from build123d import *

# Parameters (mm, degrees)
SKETCH1_R           = 5.584000144
BOSS_EXTRUDE1_DEPTH = 15
SKETCH2_R           = 2.6
CUT_EXTRUDE1_DEPTH  = 8.2
SKETCH3_R           = 2.55
CUT_EXTRUDE2_DEPTH  = 7


with BuildPart() as part:
    # Sketch1 → Boss-Extrude1 (new body)
    with BuildSketch(Plane.XY):
        with Locations((-60.533127818, -24.469533588)):
            Circle(SKETCH1_R)
    extrude(amount=BOSS_EXTRUDE1_DEPTH)

    # Sketch2 → Cut-Extrude1 (cut)
    with BuildSketch(Plane(origin=(0, 0, 0), x_dir=(-1, 0, 0), z_dir=(0, 0, -1))):
        with Locations((60.533127818, -24.469533588)):
            Circle(SKETCH2_R)
    extrude(amount=-CUT_EXTRUDE1_DEPTH, mode=Mode.SUBTRACT)

    # Sketch3 → Cut-Extrude2 (cut)
    with BuildSketch(Plane.XY.offset(15)):
        with Locations((-60.533127818, -24.469533588)):
            Circle(SKETCH3_R)
    extrude(amount=-CUT_EXTRUDE2_DEPTH, mode=Mode.SUBTRACT)


solid = part.part
Verification items for the finished model (mm, model axes). Give positions to 0.01 mm unless a question says otherwise; leave off trailing zeros. Loops run counter-clockwise (first coordinate to the right, second up) from the corner with the lowest first, then second, coordinate; pieces in that order, holes last.
1) Sectioned sample at D-D, the plane y = -19.75. Enter the section's corners in (x, z), then the cut area to 3 significant figures.
2) Draft check along Y on faces 1 (the flat face through (-58, -26, 0)), 2 (the cylindrical face through (-61.74, -29.92, 7.4)), 3 (the cylindrical face through (-58.62, -22.71, 4.04)). Enter one of: pulls with the +Y half, pulls with the -Y half, needs draft (parallel to the pull), parting line crosses it, or undercut.
3) Sectioned sample at A-A, the plane x = -59.25. Enter the section's corners in (y, z), then the cut area to 3 significant figures.
4) Depth check by flat-ended pin: pin 1 Ø3 at (x, z) = (-58.5, 2.5) entering from +Y; pin 2 Ø1 at (x, z) = (-63.5, 2.5) entering from -Y; pin 3 Ø2 at (x, z) = (-58.5, 13.5) entering from +Y; pin 4 Ø6.5 at (x, y) = (-60.53, -24.47) entering from -Z. Enter the tip coordinate at first touch or a pass-through.
5) Thickness scan on line 1 along Y through (x, z) = (-60.5, 11.25); line 2 along X through (y, z) = (-26, 3.5); line 3 along Y through (x, z) = (-61.5, 5.5). Record the ranges inside material, lowest first.
6) Sectioned sample at C-C, the plane z = 10. Enter the section's corners in (x, y).
7) Sectioned sample at B-B, the plane y = -26.5. Enter the section's corners in (x, z), then the cut area to 3 significant figures.
Answers:
1. outline: (-63.52, 0) - (-57.55, 0) - (-57.55, 15) - (-63.52, 15) - close
1. area: 89.5 mm2
2. face 1: needs draft
2. face 2: parting line crosses it
2. face 3: undercut
3. outline: (-29.9, 0) - (-26.73, 0) - (-26.73, 8.2) - (-26.67, 8.2) - (-26.67, 15) - (-29.9, 15) - close; (-22.27, 8.2) - (-22.21, 8.2) - (-22.21, 0) - (-19.03, 0) - (-19.03, 15) - (-22.27, 15) - close
3. area: 96.0 mm2
4. pin 1: stops at y = -18.91
4. pin 2: stops at y = -29.48
4. pin 3: stops at y = -18.98
4. pin 4: stops at z = 0
5. line 1: y = -30.05 to -27.02, -21.92 to -18.89
5. line 2: x = -65.9 to -62.63, -58.43 to -55.16
5. line 3: y = -29.97 to -26.88, -22.06 to -18.97
6. outline: circle Ø11.17 at (-60.53, -24.47); hole circle Ø5.1 at (-60.53, -24.47)
7. outline: (-65.73, 0) - (-62.16, 0) - (-62.16, 8.2) - (-62.08, 8.2) - (-62.08, 15) - (-65.73, 15) - close; (-58.99, 8.2) - (-58.91, 8.2) - (-58.91, 0) - (-55.33, 0) - (-55.33, 15) - (-58.99, 15) - close
7. area: 108 mm2
